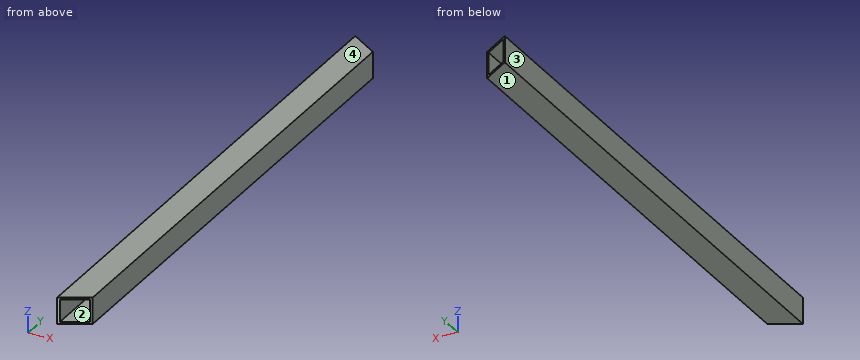
```python
from build123d import *

# Parameters (mm, degrees)
SKETCH4_W           = 13
SKETCH4_H           = 13
SKETCH4_W_2         = 11
SKETCH4_H_2         = 11
BOSS_EXTRUDE1_DEPTH = 250
CUT_EXTRUDE1_DEPTH  = 14


with BuildPart() as part:
    # Sketch4 → Boss-Extrude1 (new body)
    with BuildSketch(Plane(origin=(0, 0, 0), x_dir=(1, 0, 0), z_dir=(0, 1, 0))):
        with Locations((0.382825357, -0.030567938)):
            Rectangle(SKETCH4_W, SKETCH4_H)
        with Locations((0.382825357, -0.030567938)):
            Rectangle(SKETCH4_W_2, SKETCH4_H_2, mode=Mode.SUBTRACT)
    extrude(amount=BOSS_EXTRUDE1_DEPTH)

    # Sketch5 → Cut-Extrude1 (cut, through all)
    with BuildSketch(Plane.XY.offset(6.530567938)):
        Polygon((6.882825357, 0), (6.882825357, 7.505553499), (-6.117174643, 0), align=None)
        Polygon((6.882825357, 250), (-6.117174643, 250), (6.882825357, 242.494446501), align=None)
    extrude(amount=-CUT_EXTRUDE1_DEPTH, mode=Mode.SUBTRACT)


solid = part.part
```
Can you work these out from the model? Positions are in its coordinate system, mm. Face numbers are marked on the shaded views. Coordinates: 2 decimals unless noted, no trailing zeros. Order: outer loops, then holes, each group sorted by start corner. A loop starts at its lowest first (then second) coordinate and runs counter-clockwise, first axis right, second up.
1. If we section it at C-C (y = 123.5): Please give me the cut outline in (x, z), then the cut area to 3 significant figures.
2. If we section it at B-B (x = -1): Please give me the cut outline in (y, z), then the cut area to 3 significant figures.
3. If we section it at A-A (z = -0.5): Please give me the cut outline in (x, y).
4. I need wall thicknesses on line 1 (Z direction, x = -5, y = 29); line 2 (X direction, y = 232.5, z = -0.25); line 3 (Y direction, x = -1.25, z = 6). Which ranges of each line are inside material? Lowest first, please.
5. Thinking about a two-plate mould opening in Z: for the marked faces 1, 2, 3 and 4, which applies, +Z half, -Z half, draft (parallel to the pull), parting line (faces both ways), or undercut?
Entries:
1. outline: (-6.12, -6.47) - (6.88, -6.47) - (6.88, 6.53) - (-6.12, 6.53) - close; hole (-5.12, -5.47) - (5.88, -5.47) - (5.88, 5.53) - (-5.12, 5.53) - close
1. area: 48.0 mm2
2. outline: (2.95, -6.47) - (247.05, -6.47) - (247.05, -5.47) - (2.95, -5.47) - close; (2.95, 5.53) - (247.05, 5.53) - (247.05, 6.53) - (2.95, 6.53) - close
2. area: 488 mm2
3. outline: (-6.12, 0) - (-5.12, 0.58) - (-5.12, 249.42) - (-6.12, 250) - close; (5.88, 6.93) - (6.88, 7.51) - (6.88, 242.49) - (5.88, 243.07) - close
4. line 1: z = -6.47 to -5.47, 5.53 to 6.53
4. line 2: x = -6.12 to -5.12, 5.88 to 6.88
4. line 3: y = 2.81 to 247.19
5. face 1: -Z half
5. face 2: undercut
5. face 3: draft
5. face 4: +Z half
